Autodesk Inventor part; units mm, degrees
ref_plane "YZ Plane" through (0, 0, 0) normal (1, 0, 0) x (0, 1, 0)
ref_plane "XZ Plane" through (0, 0, 0) normal (0, 1, 0) x (-1, 0, 0)
ref_plane "XY Plane" through (0, 0, 0) normal (0, 0, 1) x (1, 0, 0)
sketch "Sketch1" plane through (0, 0, 0) normal (0, 0, 1) x (1, 0, 0)
  line L0 (0, 0) -> (50.8, 0)
  line L1 (50.8, 0) -> (50.8, 25.4)
  line L2 (50.8, 25.4) -> (0, 25.4)
  line L3 (0, 25.4) -> (0, 0)
  line L4 (25.4, 12.7) -> (25.4, 19.05)
  line L5 (25.4, 19.05) -> (38.1, 19.05)
  line L6 (38.1, 19.05) -> (12.7, 19.05)
  line L7 (12.7, 19.05) -> (12.7, 6.35)
  line L8 (12.7, 6.35) -> (38.1, 6.35)
  dimension "d0" = 50.8
  dimension "d1" = 25.4
  dimension "d2" = 6.35
  dimension "d3" = 12.7
  dimension "d4" = 25.4
  dimension "d5" = 12.7
  dimension "d6" = 25.4
extrude "Extrusion1" add sketch "Sketch1" along normal blind 6.35
hole "Hole1" at (38.1, 19.05, 0) at (38.1, 6.35, 0) at (12.7, 6.35, 0) at (12.7, 19.05, 0) direction (0, 0, 1) diameter 6.7564 end through all
fillet "Fillet1" radius 6.35 4 edges at (50.8, 25.4, 3.175) (50.8, 0, 3.175) (0, 25.4, 3.175) (0, 0, 3.175)
properties part number "WellPlateFrame-AssemblyClip"
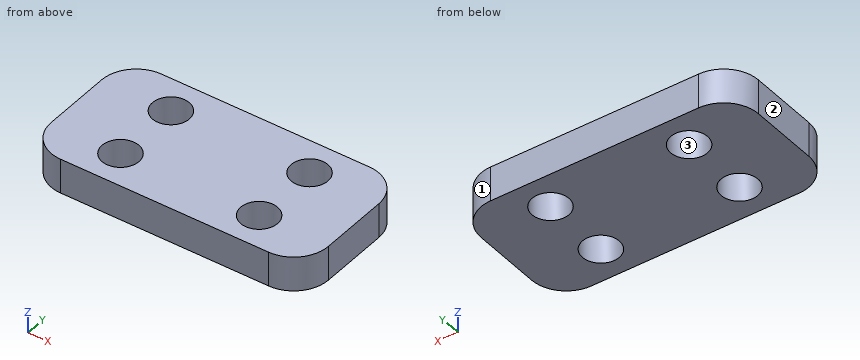
CAD build for the part. Positions are in the model's coordinates, mm. Face numbers are marked on the shaded views. Coordinates: 2 decimals unless noted, no trailing zeros. Order: outer loops, then holes, each group sorted by start corner. A loop starts at its lowest first (then second) coordinate and runs counter-clockwise, first axis right, second up. Notation, with made-up numbers: (84, -5.5) - (95, -5.5) arc R23 ccw to (95, 29.5) - close; hole circle Ø11 at (-12, 15). An arc over 180 degrees is marked (long way). Use a Markdown table: item, result. Add a question column.
(1) Saw through at D-D (x = 46). Give the cut face in (y, z), then the cut area to 3 significant figures.
(2) Saw through at C-C (z = 1). Give the cut face in (x, y), then the cut area to 3 significant figures.
(3) Saw through at B-B (y = 8.75). Give the cut face in (x, z).
(4) Pull direction X, two halves, no side cores. Call the marked faces 1, 2 and 3: +X half, -X half, draft (parallel to the pull), parting line (faces both ways), or undercut.
(5) Drill centre lines: line 1 along Y through (x, z) = (12.7, 3.5); line 2 along X through (y, z) = (19, 2.5); line 3 along X through (y, z) = (9, 4). Where is each one in solid material? Low to high. Write a range as [from, to].
(6) Saw through at A-A (x = 38.1). Give the cut face in (y, z), then the cut area to 3 significant figures.
Solved:
| question | item | result |
|---|---|---|
| 1 | outline | (0.19, 0) - (25.21, 0) - (25.21, 6.35) - (0.19, 6.35) - close |
| 1 | area | 159 mm² |
| 2 | outline | (0, 6.35) arc R6.35 ccw to (6.35, 0) - (44.45, 0) arc R6.35 ccw to (50.8, 6.35) - (50.8, 19.05) arc R6.35 ccw to (44.45, 25.4) - (6.35, 25.4) arc R6.35 ccw to (0, 19.05) - close; hole circle Ø6.76 at (12.7, 6.35); hole circle Ø6.76 at (12.7, 19.05); hole circle Ø6.76 at (38.1, 6.35); hole circle Ø6.76 at (38.1, 19.05) |
| 2 | area | 1,110 mm² |
| 3 | outline | (0, 0) - (10.32, 0) - (10.32, 6.35) - (0, 6.35) - close; (15.08, 0) - (35.72, 0) - (35.72, 6.35) - (15.08, 6.35) - close; (40.48, 0) - (50.8, 0) - (50.8, 6.35) - (40.48, 6.35) - close |
| 4 | face 1 | +X half |
| 4 | face 2 | -X half |
| 4 | face 3 | undercut |
| 5 | line 1 | y = [0, 2.97], [9.73, 15.67], [22.43, 25.4] |
| 5 | line 2 | x = [0, 9.32], [16.08, 34.72], [41.48, 50.8] |
| 5 | line 3 | x = [0, 10.6], [14.8, 36], [40.2, 50.8] |
| 6 | outline | (0, 0) - (2.97, 0) - (2.97, 6.35) - (0, 6.35) - close; (9.73, 0) - (15.67, 0) - (15.67, 6.35) - (9.73, 6.35) - close; (22.43, 0) - (25.4, 0) - (25.4, 6.35) - (22.43, 6.35) - close |
| 6 | area | 75.5 mm² |
